Read the model definition and answer for the solid it produces. Units are mm, in the model's axes. A direction names the side the tool comes from. Coordinates: 2 decimals unless noted, no trailing zeros. Loops run counter-clockwise (first coordinate to the right, second up) from the corner with the lowest first, then second, coordinate; pieces in that order, holes last. Notation, with made-up numbers: (-14, 61) -> (-7, 61) arc R11 cw to (-7, 72) -> close; hole circle Ø1 at (17.5, 52.25). An arc over 180 degrees is marked (long way). Answer as a JSON object with one key per item and string values. Group by question number.
1) Flat-ended cylindrical pins translate along their axes: P1, Ø20, axis at y = 1.5, z = 8.5, coming from the -X side; P2, Ø1, axis at x = -5, z = 0.5, coming from the -Y side; P3, Ø1, axis at x = -6, z = -5, coming from the +Y side; P4, Ø3, axis at x = -5.5, y = 15.5, coming from the -Z side. Find the tip coordinate at first contact, or state that the pin passes through.
2) Which of the six approach directions +Z, -Z, +X, -X, +Y, -Y give full straight-line access (tool end or side, diameter ignored) to faces 5 (the face through (-5.96, 10.34, -14.99)), 6 (the face through (-2.514, -4.336, -19.524)), 7 (the face through (-0.021, -13.887, -10.648))?
3) Section B-B, the plane y = 0 is taken. Give the vertices of the cut face in (x, z), plus the area to 3 significant figures.
4) Section A-A, the plane z = -10 is taken. Give the vertices of the cut face in (x, y).
5) Consider probe 1 along Z at (x, y) = (1.25, 0); probe 2 along X at (y, z) = (-12, -15.5); probe 3 along X at (y, z) = (6.5, -16). Determine where each line is inside the solid, lowest interval first. Write a range as [from, to].
6) Determine the mould class of faces 1 (the face through (-5.965, -2.195, -11.203)), 2 (the face through (-5.96, -11.82, -0.96)), 3 (the face through (3.5, 0, 0)), 4 (the face through (-5.965, -0.358, -24.835)) for opening direction Y: released by +Y, released by -Y, zero draft, split by the parting line, or undercut.
7) Section C-C, the plane x = -4.5 is taken. Give the vertices of the cut face in (y, z).
8) Section D-D, the plane y = -5.5 is taken. Give the vertices of the cut face in (x, z).
from build123d import *

# Parameters (mm, degrees)
BOSS_EXTRUDE1_DEPTH = 5
SKETCH4_R           = 2.5
CUT_EXTRUDE1_DEPTH  = 8


with BuildPart() as part:
    # Sketch1 → Revolve1 (revolve)
    with BuildSketch(Plane.XY):
        Polygon((-3.5, 20), (-3.5, 0), (3.5, 0), (3.5, 20), (1.5, 20), (1.5, 17.5), (-1.5, 17.5), (-1.5, 20), align=None)
    revolve(axis=Axis((-3.5, 0, 0), (1, 0, 0)))

    # Sketch3 → Boss-Extrude1 (add)
    with BuildSketch(Plane.ZY.offset(3.5)):
        with BuildLine():
            Line((-10.907816743, 18.773009049), (-19.189724736, 1.673009049))
            Line((-19.189724736, 1.673009049), (-2.989724736, -6.173009049))
            Line((-2.989724736, -6.173009049), (5.292183257, 10.926990951))
            Line((5.292183257, 10.926990951), (10.692183257, 8.311651585))
            Line((10.692183257, 8.311651585), (2.410275264, -8.788348415))
            ThreePointArc((2.410275264, -8.788348415), (-1.020672318, -11.840709868), (-5.605064102, -11.573009049))
            Line((-5.605064102, -11.573009049), (-21.805064102, -3.726990951))
            ThreePointArc((-21.805064102, -3.726990951), (-24.857425555, -0.296043368), (-24.589724736, 4.288348415))
            Line((-24.589724736, 4.288348415), (-16.307816743, 21.388348415))
            Line((-16.307816743, 21.388348415), (-10.907816743, 18.773009049))
        make_face()
    extrude(amount=BOSS_EXTRUDE1_DEPTH)

    # Sketch4 → Cut-Extrude1 (cut, through all)
    with BuildSketch(Plane.ZY.offset(3.5)):
        with Locations((-10, 0)):
            Circle(SKETCH4_R)
    extrude(amount=-CUT_EXTRUDE1_DEPTH, mode=Mode.SUBTRACT)


solid = part.part
Determined:
{
 "1": {"P1": "x = -8.5", "P2": "y = -11.38", "P3": "y = -4.96", "P4": "z = -19.89"},
 "2": {"face 5": "-X", "face 6": "+X", "face 7": "none"},
 "3": {"outline": "(-8.5, -24.95) -> (-3.5, -24.95) -> (-3.5, -20) -> (-1.5, -20) -> (-1.5, -17.5) -> (1.5, -17.5) -> (1.5, -20) -> (3.5, -20) -> (3.5, -12.5) -> (-3.5, -12.5) -> (-3.5, -15.74) -> (-8.5, -15.74) -> close; (-8.5, 0) -> (-3.5, 0) -> (-3.5, -7.5) -> (3.5, -7.5) -> (3.5, 20) -> (1.5, 20) -> (1.5, 17.5) -> (-1.5, 17.5) -> (-1.5, 20) -> (-3.5, 20) -> (-3.5, 6.67) -> (-8.5, 6.67) -> close", "area": "309 mm²"},
 "4": {"outline": "(-8.5, -9.44) -> (-3.5, -9.44) -> (-3.5, -17.32) -> (-1.5, -17.32) -> (-1.5, -14.36) -> (1.5, -14.36) -> (1.5, -17.32) -> (3.5, -17.32) -> (3.5, -2.5) -> (-3.5, -2.5) -> (-3.5, -2.78) -> (-8.5, -2.78) -> close; (-3.5, 2.5) -> (3.5, 2.5) -> (3.5, 17.32) -> (1.5, 17.32) -> (1.5, 14.36) -> (-1.5, 14.36) -> (-1.5, 17.32) -> (-3.5, 17.32) -> close"},
 "5": {"probe 1": "[-17.5, -12.5], [-7.5, 17.5]", "probe 2": "[-3.5, -1.5], [1.5, 3.5]", "probe 3": "[-3.5, 3.5]"},
 "6": {"face 1": "undercut", "face 2": "released by -Y", "face 3": "zero draft", "face 4": "split by the parting line"},
 "7": {"outline": "(-11.57, -5.61) -> (-3.73, -21.81) arc R6 ccw to (4.29, -24.59) -> (21.39, -16.31) -> (18.77, -10.91) -> (1.67, -19.19) -> (-6.17, -2.99) -> (10.93, 5.29) -> (8.31, 10.69) -> (-8.79, 2.41) arc R6 ccw to start"},
 "8": {"outline": "(-8.5, -18.14) -> (-3.5, -18.14) -> (-3.5, -19.23) -> (-1.5, -19.23) -> (-1.5, -16.61) -> (1.5, -16.61) -> (1.5, -19.23) -> (3.5, -19.23) -> (3.5, 19.23) -> (1.5, 19.23) -> (1.5, 16.61) -> (-1.5, 16.61) -> (-1.5, 19.23) -> (-3.5, 19.23) -> (-3.5, 4) -> (-8.5, 4) -> (-8.5, -2.66) -> (-3.5, -2.66) -> (-3.5, -4.38) -> (-8.5, -4.38) -> close"}
}
